Here's how the part is built. I have some questions about the finished solid (model axes, mm). A direction names the side the tool comes from. Coordinates: 2 decimals unless noted, no trailing zeros. Order: outer loops, then holes, each group sorted by start corner. A loop starts at its lowest first (then second) coordinate and runs counter-clockwise, first axis right, second up. Notation, with made-up numbers: M -8.75,24.25 L 46.25,24.25 A21 ccw 46.25,29.25 Z; hole C 68.5,1 d4. An arc over 180 degrees is marked long. One line per question, with ' | ' between items. Start each with the question number.
```python
from build123d import *

# Parameters (mm, degrees)
BOX008_W       = 10
BOX008_H       = 6
BOX008_DEPTH   = 1.5
BOX009_W       = 10
BOX009_H       = 6
BOX009_DEPTH   = 1.5
BOX010_W       = 6
BOX010_H       = 10
BOX010_DEPTH   = 1.5
BOX011_W       = 6
BOX011_H       = 10
BOX011_DEPTH   = 1.5
BOX007_W       = 6
BOX007_H       = 17.5
BOX007_DEPTH   = 6
FILLET_R       = 1
BOX006_W       = 17.5
BOX006_H       = 6
BOX006_DEPTH   = 6
FILLET001_R    = 1
CYLINDER_R     = 6
CYLINDER_DEPTH = 0.5


with BuildPart() as cube:
    # Box008 → Box008 (new body)
    with BuildSketch(Plane(origin=(4.5, -3, 0), x_dir=(1, 0, 0), z_dir=(0, 0, 1))):
        with Locations((5, 3)):
            Rectangle(BOX008_W, BOX008_H)
    extrude(amount=BOX008_DEPTH)


with BuildPart() as cube001:
    # Box009 → Box009 (new body)
    with BuildSketch(Plane(origin=(-14.5, -3, 0), x_dir=(1, 0, 0), z_dir=(0, 0, 1))):
        with Locations((5, 3)):
            Rectangle(BOX009_W, BOX009_H)
    extrude(amount=BOX009_DEPTH)


with BuildPart() as cube002:
    # Box010 → Box010 (new body)
    with BuildSketch(Plane(origin=(-3, 4.5, 0), x_dir=(1, 0, 0), z_dir=(0, 0, 1))):
        with Locations((3, 5)):
            Rectangle(BOX010_W, BOX010_H)
    extrude(amount=BOX010_DEPTH)


with BuildPart() as cube003:
    # Box011 → Box011 (new body)
    with BuildSketch(Plane(origin=(-3, -14.5, 0), x_dir=(1, 0, 0), z_dir=(0, 0, 1))):
        with Locations((3, 5)):
            Rectangle(BOX011_W, BOX011_H)
    extrude(amount=BOX011_DEPTH)


with BuildPart() as fillet_body:
    # Box007 → Box007 (new body)
    with BuildSketch(Plane(origin=(-3, -8.75, 0), x_dir=(1, 0, 0), z_dir=(0, 0, 1))):
        with Locations((3, 8.75)):
            Rectangle(BOX007_W, BOX007_H)
    extrude(amount=BOX007_DEPTH)

    # Fillet
    fillet_edges = [fillet_body.edges().sort_by_distance(p)[0] for p in [
        (-3, 0, 6),
        (3, 0, 6),
        (0, -8.75, 6),
        (0, 8.75, 6),
    ]]
    fillet(fillet_edges, radius=FILLET_R)


with BuildPart() as fusion:
    # Box006 → Box006 (new body)
    with BuildSketch(Plane(origin=(-8.75, -3, 0), x_dir=(1, 0, 0), z_dir=(0, 0, 1))):
        with Locations((8.75, 3)):
            Rectangle(BOX006_W, BOX006_H)
    extrude(amount=BOX006_DEPTH)

    # Fillet001
    fillet001_edges = [fusion.edges().sort_by_distance(p)[0] for p in [
        (-8.75, 0, 6),
        (8.75, 0, 6),
        (0, -3, 6),
        (0, 3, 6),
    ]]
    fillet(fillet001_edges, radius=FILLET001_R)

    # Fusion: union Fillet body
    add(fillet_body.part)


with BuildPart() as cut003:
    # Cylinder → Cylinder (new body)
    with BuildSketch(Plane.XY):
        Circle(CYLINDER_R)
    extrude(amount=CYLINDER_DEPTH)

    # Fusion001: union Fusion
    add(fusion.part)

    # Cut: cut Cube003
    add(cube003.part, mode=Mode.SUBTRACT)

    # Cut001: cut Cube002
    add(cube002.part, mode=Mode.SUBTRACT)

    # Cut002: cut Cube001
    add(cube001.part, mode=Mode.SUBTRACT)

    # Cut003: cut Cube
    add(cube.part, mode=Mode.SUBTRACT)


solid = cut003.part
```
1. Will these pins go through, and if not, where does the flat tip stop? pin 1 (3 mm diameter, centred on y = -6, z = 1, fed in from -X); pin 2 (1.8 mm diameter, centred on x = 4.5, y = -4, fed in from +Z); pin 3 (0.8 mm diameter, centred on y = 0.5, z = 0.5, fed in from +X).
2. Imagine slicing it at C-C (z = 2.25). List the corners of the cut face in (x, y) for me, then the cut area to 3 significant figures.
3. Imagine slicing it at A-A (x = 0.5). List the corners of the cut face in (y, z) for me, then the cut area to 3 significant figures.
4. We'd pull the mould along Y, two halves only. Please class faces 6 (the face through (4.227, -4.258, 0.246)), 7 (the face through (-4.5, 0, 1)), 8 (the face through (8.465, 0.042, 5.699)): released by +Y, released by -Y, zero draft, split by the parting line, or undercut.
5. Imagine slicing it at D-D (x = 6.75). List the corners of the cut face in (y, z) for me, then the cut area to 3 significant figures.
6. Which directions (+Z, -Z, +X, -X, +Y, -Y) give clear straight access to the entire face, cutting with the end or side of a thin tool? Please do faces 1 (the face through (0, -7, 1.5)), 2 (the face through (6, -3, 3)), 3 (the face through (-4, 4, 0.5)), 4 (the face through (-6, -3, 3)), 5 (the face through (3, 6, 3)).
7. I need wall thicknesses on line 1 (X direction, y = 3.5, z = 0.75); line 2 (X direction, y = 2.5, z = 1.4). Which ranges of each line are inside material? Lowest first, please.
Entries:
1) pin 1: x = -3.87 | pin 2: z = 0.5 | pin 3: x = 4.5
2) outline: M -8.75,-3 L -3,-3 L -3,-8.75 L 3,-8.75 L 3,-3 L 8.75,-3 L 8.75,3 L 3,3 L 3,8.75 L -3,8.75 L -3,3 L -8.75,3 Z | area: 174 mm²
3) outline: M -8.75,1.5 L -4.5,1.5 L -4.5,0 L 4.5,0 L 4.5,1.5 L 8.75,1.5 L 8.75,5 A1 ccw 7.75,6 L -7.75,6 A1 ccw -8.75,5 Z | area: 91.8 mm²
4) face 6: released by -Y | face 7: undercut | face 8: zero draft
5) outline: M -3,1.5 L 3,1.5 L 3,5 A1 ccw 2,6 L -2,6 A1 ccw -3,5 Z | area: 26.6 mm²
6) face 1: -Z, +X, -X, -Y | face 2: +Z, +X, -Y | face 3: +Z, -X, +Y | face 4: +Z, -X, -Y | face 5: +Z, +X, +Y
7) line 1: -3 to 3 | line 2: -4.5 to 4.5
